```python
from build123d import *

# Parameters (mm, degrees)
SKETCH_1_W          = 12
SKETCH_1_H          = 15
SKETCH_1_R          = 1.75
EXTRUDE_1_DEPTH     = 4
SKETCH_2_W          = 16
SKETCH_2_H          = 15
SKETCH_2_R          = 1.75
EXTRUDE_2_DEPTH     = 4
FILLET_1_R          = 2
SKETCH_3_W          = 2
SKETCH_3_H          = 15
CUT_EXTRUDE_1_DEPTH = 4
SKETCH_4_W          = 2
SKETCH_4_H          = 15
CUT_EXTRUDE_2_DEPTH = 4


with BuildPart() as part:
    # 草图1 → 凸台-拉伸1 (new body)
    with BuildSketch(Plane.XY):
        Rectangle(SKETCH_1_W, SKETCH_1_H)
        with Locations((2, 0)):
            Circle(SKETCH_1_R, mode=Mode.SUBTRACT)
    extrude(amount=EXTRUDE_1_DEPTH)

    # 草图2 → 凸台-拉伸2 (add)
    with BuildSketch(Plane(origin=(6, 0, 0), x_dir=(0, 0, -1), z_dir=(1, 0, 0))):
        with Locations((4, 0)):
            Rectangle(SKETCH_2_W, SKETCH_2_H)
        with Locations((4, 0)):
            Circle(SKETCH_2_R, mode=Mode.SUBTRACT)
    extrude(amount=EXTRUDE_2_DEPTH)

    # 圆角1
    fillet_1_edges = [part.edges().sort_by_distance(p)[0] for p in [
        (6, 0, 0),
    ]]
    fillet(fillet_1_edges, radius=FILLET_1_R)

    # 草图3 → 切除-拉伸1 (cut)
    with BuildSketch(Plane.ZY.offset(-6)):
        with Locations((-11, 0)):
            Rectangle(SKETCH_3_W, SKETCH_3_H)
    extrude(amount=-CUT_EXTRUDE_1_DEPTH, mode=Mode.SUBTRACT)

    # 草图4 → 切除-拉伸2 (cut)
    with BuildSketch(Plane(origin=(0, 0, 0), x_dir=(-1, 0, 0), z_dir=(0, 0, -1))):
        with Locations((5, 0)):
            Rectangle(SKETCH_4_W, SKETCH_4_H)
    extrude(amount=-CUT_EXTRUDE_2_DEPTH, mode=Mode.SUBTRACT)


solid = part.part
```
Could you check a few things on this model? Use its own coordinates, in mm. A direction names the side the tool comes from. Coordinates: 2 decimals unless noted, no trailing zeros. Write each loop counter-clockwise with the first axis right and the second up, starting at its lowest first coordinate (ties: lowest second). Pieces come first, ordered by that corner, then holes. Notation, with made-up numbers: (33, 22.5) -> (74, 22.5) arc R21 ccw to (74, 37.5) -> close; hole circle Ø9 at (17.25, -21). An arc over 180 degrees is marked (long way). Return JSON: item names as keys, results as strings.
(1) I need wall thicknesses on L1, parallel to Y at x = 7.5, z = -4; L2, parallel to X at y = 4.5, z = -7.5; L3, parallel to Z at x = 0.5, y = -5.5. Which ranges of each line are inside material? Lowest first, please.
Numbers:
{"L1": "y = -7.5 to -1.75, 1.75 to 7.5", "L2": "x = 6 to 10", "L3": "z = 0 to 4"}
(2) Imagine slicing it at B-B, the plane z = -4. Please give me the cut outline in (x, y), then the cut area to 3 significant figures.
Numbers:
{"outline": "(6, -7.5) -> (10, -7.5) -> (10, -1.75) -> (6, -1.75) -> close; (6, 1.75) -> (10, 1.75) -> (10, 7.5) -> (6, 7.5) -> close", "area": "46.0 mm2"}
(3) I'm going to push flat-ended pins straight in: pin 1 (1 mm diameter, centred on x = 1, y = 4, fed in from -Z); pin 2 (6.5 mm diameter, centred on y = -1.5, z = -4, fed in from -X). Where does each tip first touch, or does it pass through?
Numbers:
{"pin 1": "stops at z = 0", "pin 2": "stops at x = 5.56"}
(4) We'd pull the mould along X, two halves only. Please class faces 1 (the cylindrical face through (3.669, 0.526, 1.972)), 2 (the flat face through (6, 0, -6)), 3 (the flat face through (8, 0, -10)): +X half, -X half, draft (parallel to the pull), parting line (faces both ways), or undercut.
Numbers:
{"face 1": "undercut", "face 2": "-X half", "face 3": "draft"}
(5) Imagine slicing it at C-C, the plane y = 0. Please give me the cut outline in (x, z).
Numbers:
{"outline": "(-4, 0) -> (0.25, 0) -> (0.25, 4) -> (-4, 4) -> close; (3.75, 0) -> (4, 0) arc R2 cw to (6, -2) -> (6, -2.25) -> (10, -2.25) -> (10, 4) -> (3.75, 4) -> close; (6, -10) -> (10, -10) -> (10, -5.75) -> (6, -5.75) -> close"}
(6) Imagine slicing it at A-A, the plane x = 2. Please give me the cut outline in (y, z), then the cut area to 3 significant figures.
Numbers:
{"outline": "(-7.5, 0) -> (-1.75, 0) -> (-1.75, 4) -> (-7.5, 4) -> close; (1.75, 0) -> (7.5, 0) -> (7.5, 4) -> (1.75, 4) -> close", "area": "46.0 mm2"}
(7) Which directions (+Z, -Z, +X, -X, +Y, -Y) give clear straight access to the entire face, cutting with the end or side of a thin tool? Please do faces 4 (the cylindrical face through (7.97, 0.08, -2.25)), 5 (the flat face through (0, 0, 0)).
Numbers:
{"face 4": "+X, -X", "face 5": "-Z, -X, +Y, -Y"}
(8) Imagine slicing it at D-D, the plane y = -6.5. Please give me the cut outline in (x, z).
Numbers:
{"outline": "(-4, 0) -> (4, 0) arc R2 cw to (6, -2) -> (6, -10) -> (10, -10) -> (10, 4) -> (-4, 4) -> close"}
